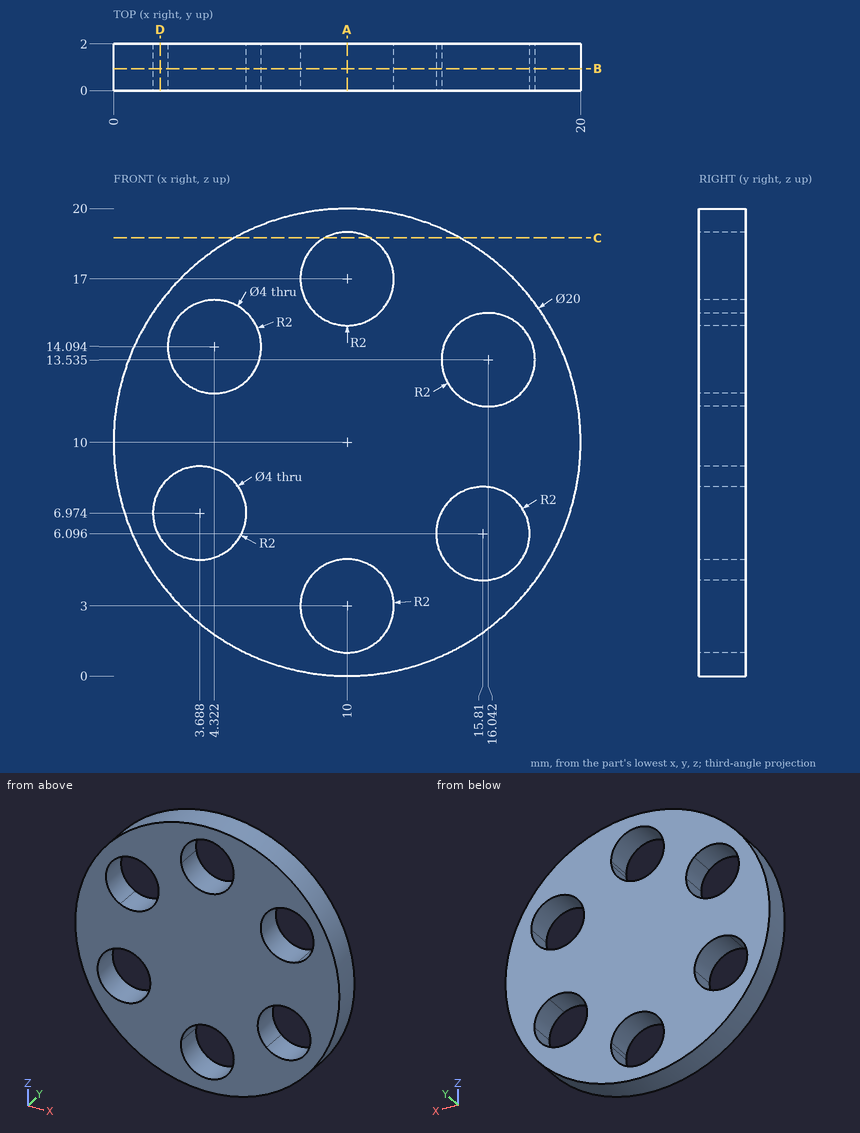
Verification items for this drawing (mm, ordinates from the low corner). Give positions to 0.01 mm unless a question says otherwise; leave off trailing zeros. Write each loop counter-clockwise with the first axis right and the second up, starting at its lowest first coordinate (ties: lowest second). Pieces come first, ordered by that corner, then holes.
1) Thickness scan on line 1 (Z direction, x = 5, y = 1.7) (1 decimal); line 2 (Z direction, x = 5.25, y = 0.9) (1 decimal); line 3 (X direction, y = 1, z = 7) (1 decimal). Record the ranges inside material, lowest first.
Values follow:
line 1: z = 1.3 to 5.5, 8.5 to 12.2, 16 to 18.7
line 2: z = 1.2 to 5.7, 8.2 to 12.3, 15.9 to 18.8
line 3: x = 0.5 to 1.7, 5.7 to 14, 17.6 to 19.5
2) Cross-section at C-C (z = 18.75). Record the boundary of the cut face in (x, y), plus the area to 3 significant figures.
Values follow:
outline: (5.16, 0) - (9.03, 0) - (9.03, 2) - (5.16, 2) - close; (10.97, 0) - (14.84, 0) - (14.84, 2) - (10.97, 2) - close
area: 15.5 mm2
3) Cross-section at A-A (x = 10). Record the boundary of the cut face in (y, z), plus the area to 3 significant figures.
Values follow:
outline: (0, 0) - (2, 0) - (2, 1) - (0, 1) - close; (0, 5) - (2, 5) - (2, 15) - (0, 15) - close; (0, 19) - (2, 19) - (2, 20) - (0, 20) - close
area: 24.0 mm2
4) Cross-section at D-D (x = 2). Record the boundary of the cut face in (y, z), plus the area to 3 significant figures.
Values follow:
outline: (0, 4) - (2, 4) - (2, 5.9) - (0, 5.9) - close; (0, 8.05) - (2, 8.05) - (2, 16) - (0, 16) - close
area: 19.7 mm2
5) Go/stop test with a flat-tipped pin: pin 1 Ø4.5 at (x, z) = (4.32, 14.09) entering from +Y. Record where the tip stops, or that it passes through.
Values follow:
pin 1: stops at y = 2
6) Cross-section at B-B (y = 0.95). Record the boundary of the cut face in (x, z) (1 decimal), plus the area to 3 significant figures.
Values follow:
outline: circle Ø20 at (10, 10); hole circle Ø4 at (3.7, 7); hole circle Ø4 at (4.3, 14.1); hole circle Ø4 at (10, 3); hole circle Ø4 at (10, 17); hole circle Ø4 at (15.8, 6.1); hole circle Ø4 at (16, 13.5)
area: 239 mm2
